Read the model definition and answer for the solid it produces. Units are mm, in the model's axes. Coordinates: 2 decimals unless noted, no trailing zeros. Loops run counter-clockwise (first coordinate to the right, second up) from the corner with the lowest first, then second, coordinate; pieces in that order, holes last. Notation, with made-up numbers: M 17.25,82.25 L 41.25,82.25 A12 ccw 41.25,98.25 Z; hole C 56.25,27.5 d11. An arc over 180 degrees is marked long. One line per item, written item: value. Start each with the question number.
1. The part is cut by section A-A (x = 0). Write down the section's boundary in (y, z).
2. The part is cut by section D-D (z = 3.9). State how many separate pieces and enclosed holes the cut face has, then the cut area to 3 significant figures.
3. The part is cut by section B-B (y = -6). Write down the section's boundary in (x, z), then the cut area to 3 significant figures.
4. Flat-ended cylindrical pins translate along their axes: pin 1 (2.5 mm diameter, centred on x = 41.8, y = -47.658, fed in from -Z); pin 2 (1 mm diameter, centred on y = 30.5, z = 1.5, fed in from +X); pin 3 (2 mm diameter, centred on y = 6, z = 5, fed in from +X); pin 4 (2 mm diameter, centred on y = 6.5, z = 5, fed in from -X). Find the tip coordinate at first contact, or state that the pin passes through.
5. Consider probe 1 along Y at (x, z) = (0.5, 4.75); probe 2 along Y at (x, z) = (-9, 0.4); probe 3 along X at (y, z) = (-13.5, 4). Determine where each line is inside the solid, lowest interval first.
6. The part is cut by section C-C (x = -18.5). Write down the section's boundary in (y, z).
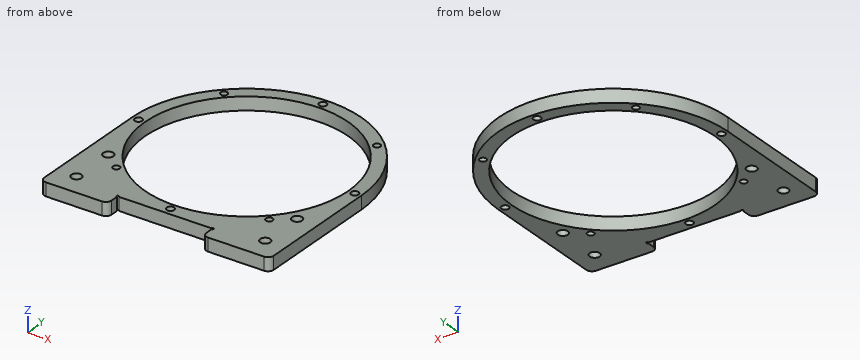
```python
from build123d import *

# Parameters (mm, degrees)
SKETCH1_R           = 2.25
SKETCH1_R_2         = 44.958
SKETCH1_R_3         = 1.65
SKETCH1_R_4         = 1.5
BOSS_EXTRUDE1_DEPTH = 5.842
SKETCH2_W           = 42
SKETCH2_H           = 6.35
CUT_EXTRUDE1_DEPTH  = 78.066295668
SKETCH3_R           = 0.5
CUT_EXTRUDE2_DEPTH  = 78.066295668
FILLET1_R           = 2.54


with BuildPart() as part:
    # Sketch1 → Boss-Extrude1 (new body)
    with BuildSketch(Plane.XY):
        with BuildLine():
            Line((-50.8, 0), (-50.8, -57.658))
            Line((-50.8, -57.658), (50.8, -57.658))
            Line((50.8, -57.658), (50.8, 0))
            ThreePointArc((50.8, 0), (0, 50.8), (-50.8, 0))
        make_face()
        with Locations((41.8, -47.658)):
            Circle(SKETCH1_R, mode=Mode.SUBTRACT)
        Circle(SKETCH1_R_2, mode=Mode.SUBTRACT)
        with Locations((-47.879, 0)):
            Circle(SKETCH1_R_3, mode=Mode.SUBTRACT)
        with Locations((0, 47.879)):
            Circle(SKETCH1_R_3, mode=Mode.SUBTRACT)
        with Locations((41.8, -27.658)):
            Circle(SKETCH1_R, mode=Mode.SUBTRACT)
        with Locations((47.879, 0)):
            Circle(SKETCH1_R_3, mode=Mode.SUBTRACT)
        with Locations((0, -47.879)):
            Circle(SKETCH1_R_3, mode=Mode.SUBTRACT)
        with Locations((-41.8, -27.658)):
            Circle(SKETCH1_R, mode=Mode.SUBTRACT)
        with Locations((-33.855565576, 33.855565576)):
            Circle(SKETCH1_R_4, mode=Mode.SUBTRACT)
        with Locations((33.855565576, 33.855565576)):
            Circle(SKETCH1_R_4, mode=Mode.SUBTRACT)
        with Locations((33.855565576, -33.855565576)):
            Circle(SKETCH1_R_4, mode=Mode.SUBTRACT)
        with Locations((-33.855565576, -33.855565576)):
            Circle(SKETCH1_R_4, mode=Mode.SUBTRACT)
        with Locations((-41.8, -47.658)):
            Circle(SKETCH1_R, mode=Mode.SUBTRACT)
    extrude(amount=BOSS_EXTRUDE1_DEPTH)

    # Sketch2 → Cut-Extrude1 (cut, through all)
    with BuildSketch(Plane.XY.offset(5.842)):
        with Locations((0, -54.483)):
            Rectangle(SKETCH2_W, SKETCH2_H)
    extrude(amount=-CUT_EXTRUDE1_DEPTH, mode=Mode.SUBTRACT)

    # Sketch3 → Cut-Extrude2 (cut, through all)
    with BuildSketch(Plane.XY.offset(5.842)):
        with Locations((-21, -51.308)):
            Circle(SKETCH3_R)
        with Locations((21, -51.308)):
            Circle(SKETCH3_R)
    extrude(amount=-CUT_EXTRUDE2_DEPTH, mode=Mode.SUBTRACT)

    # Fillet1
    fillet1_edges = [part.edges().sort_by_distance(p)[0] for p in [
        (50.8, -57.658, 2.921),
        (-50.8, -57.658, 2.921),
        (-21, -57.658, 2.921),
        (21, -57.658, 2.921),
    ]]
    fillet(fillet1_edges, radius=FILLET1_R)


solid = part.part
```
Answer block:
1. outline: M -51.31,0 L -49.53,0 L -49.53,5.84 L -51.31,5.84 Z; M -46.23,0 L -44.96,0 L -44.96,5.84 L -46.23,5.84 Z; M 44.96,0 L 46.23,0 L 46.23,5.84 L 44.96,5.84 Z; M 49.53,0 L 50.8,0 L 50.8,5.84 L 49.53,5.84 Z
2. separate pieces: 1
2. enclosed holes: 13
2. area: 3,160 mm2
3. outline: M -50.8,0 L -44.56,0 L -44.56,5.84 L -50.8,5.84 Z; M 44.56,0 L 50.8,0 L 50.8,5.84 L 44.56,5.84 Z
3. area: 73.0 mm2
4. pin 1: passes through
4. pin 2: stops at x = 41
4. pin 3: stops at x = 50.55
4. pin 4: stops at x = -50.5
5. probe 1: y = -51.31 to -49.45, -46.31 to -44.96, 44.96 to 46.31, 49.45 to 50.8
5. probe 2: y = -51.31 to -44.05, 44.05 to 50
5. probe 3: x = -50.8 to -42.88, 42.88 to 50.8
6. outline: M -51.31,0 L -40.98,0 L -40.98,5.84 L -51.31,5.84 Z; M 40.98,0 L 47.31,0 L 47.31,5.84 L 40.98,5.84 Z
